```python
from build123d import *

# Parameters (mm, degrees)
RESSALTO_EXTRUS_O1_DEPTH = 3
FURO_COM_FOLGA_DE_M61_D  = 6.6
CORTE_EXTRUS_O1_DEPTH    = 101.321862822


with BuildPart() as part:
    # Esboço1 → Ressalto-extrusão1 (new body)
    with BuildSketch(Plane.XY):
        Polygon((0, 0), (0, 60), (30, 60), (80.345977871, 0), align=None)
    extrude(amount=RESSALTO_EXTRUS_O1_DEPTH)

    # Furo com folga de M61 (through all)
    with Locations(Plane.XY.offset(3)):
        with Locations((15.913142528, 21.022225211), (12.030856852, 35.511112606), (8.148571175, 50)):
            Hole(FURO_COM_FOLGA_DE_M61_D / 2)

    # Esboço4 → Corte-extrusão1 (cut, through all)
    with BuildSketch(Plane.XY.offset(3)):
        Polygon((0, 36), (10, 16), (72, 0), (0, 0), align=None)
    extrude(amount=-CORTE_EXTRUS_O1_DEPTH, mode=Mode.SUBTRACT)


solid = part.part
```
Input: part model. Units: mm. Frame: model coordinates. Give positions to 0.01 mm unless a question says otherwise; leave off trailing zeros. Loops run counter-clockwise (first coordinate to the right, second up) from the corner with the lowest first, then second, coordinate; pieces in that order, holes last. Notation, with made-up numbers: (24, 48) -> (79, 48) arc R12 ccw to (79, 56) -> close; hole circle Ø9 at (56.25, 73.25). An arc over 180 degrees is marked (long way). Use a Markdown table: item, result.
Q1. Ray query, probe 1 along X at (y, z) = (22, 1.8); probe 2 along X at (y, z) = (35.5, 0.45); probe 3 along Y at (x, z) = (27, 0.7). Return the intervals inside material, ascending. Write a range as from..to.
Entries:
| item | result |
|---|---|
| probe 1 | x = 7..12.76, 19.06..61.89 |
| probe 2 | x = 0.25..8.73, 15.33..50.56 |
| probe 3 | y = 11.61..60 |
Q2. Section query A-A, the plane y = 50. Return the cut outline in (x, z).
Entries:
| item | result |
|---|---|
| outline | (0, 0) -> (4.85, 0) -> (4.85, 3) -> (0, 3) -> close; (11.45, 0) -> (38.39, 0) -> (38.39, 3) -> (11.45, 3) -> close |
Q3. Section query C-C, the plane y = 28. Return the cut outline in (x, z).
Entries:
| item | result |
|---|---|
| outline | (4, 0) -> (56.85, 0) -> (56.85, 3) -> (4, 3) -> close |
Q4. Pull-direction query (X, two-part tool) for faces 1 (the flat face through (0, 48, 1)), 2 (the cylindrical face through (6.4, 52.8, 1.5)), 3 (the flat face through (32, 30, 0)); classes: pulls with the +X half, pulls with the -X half, needs draft (parallel to the pull), parting line crosses it, or undercut.
Entries:
| item | result |
|---|---|
| face 1 | pulls with the -X half |
| face 2 | undercut |
| face 3 | needs draft |
Q5. First-contact query: P1, Ø1, axis at y = 31.5, z = 0.5, coming from the +X side. Flat tip, straight axial feed; report the tip coordinate or a pass-through.
Entries:
| item | result |
|---|---|
| P1 | stops at x = 54.33 |
Q6. Section query D-D, the plane x = 74. Return the cut outline in (y, z), plus the area to 3 significant figures.
Entries:
| item | result |
|---|---|
| outline | (0, 0) -> (7.56, 0) -> (7.56, 3) -> (0, 3) -> close |
| area | 22.7 mm² |
Q7. Section query B-B, the plane z = 0.85. Return the cut outline in (x, y), plus the area to 3 significant figures.
Entries:
| item | result |
|---|---|
| outline | (0, 36) -> (10, 16) -> (72, 0) -> (80.35, 0) -> (30, 60) -> (0, 60) -> close; hole circle Ø6.6 at (8.15, 50); hole circle Ø6.6 at (12.03, 35.51); hole circle Ø6.6 at (15.91, 21.02) |
| area | 2,450 mm² |
